Could you check a few things on this model? Use its own coordinates, in mm. A direction names the side the tool comes from. Give positions to 0.01 mm unless a question says otherwise; leave off trailing zeros. Order: outer loops, then holes, each group sorted by start corner. A loop starts at its lowest first (then second) coordinate and runs counter-clockwise, first axis right, second up.
(1) Imagine slicing it at B-B, the plane x = 6. Write out the boundary of the cut face in (y, z).
(2) If I drill on probe 1 along Y at (x, z) = (4.25, 0); probe 2 along Y at (x, z) = (10.3, 0) (3 decimals); probe 3 along X at (y, z) = (0.25, 5), over which ranges is the centre line in solid material (lowest first)?
(3) If we mould it in two halves opening along Z, with no side actions, what happens to faces 4 (the flat face through (10, 2, 2)), 5 (the flat face through (10.8, -5, -5)), 6 (the cylindrical face through (3.94, 1.1, -3.48))? For each: released by +Z, released by -Z, zero draft, split by the parting line, or undercut.
(4) Will these pins go through, and if not, where does the flat tip stop? pin 1 (2 mm diameter, centred on x = 9, y = -6, fed in from -Z); pin 2 (3 mm diameter, centred on x = 1, y = -4.5, fed in from -Z); pin 3 (2 mm diameter, centred on x = 4, y = -3.5, fed in from -Z); pin 4 (3.5 mm diameter, centred on y = 0, z = 0, fed in from +X).
(5) Imagine slicing it at A-A, the plane z = 0. Write out the boundary of the cut face in (x, y) (3 decimals).
(6) On a 3-axis mill with a long thin cutter (end or side, diameter ignored), from which of +Z, -Z, +X, -X, +Y, -Y can I reach the whole of each face in a straight line? I mean faces 1 (the flat face through (8, 0, -4)), 2 (the cylindrical face through (4.93, 0.631, -2.003)), 3 (the cylindrical face through (9.44, 8.38, 3.71)). Say none if no direction works.
from build123d import *

# Parameters (mm, degrees)
SKETCH3_R           = 3.65
SKETCH3_R_2         = 2.1
BOSS_EXTRUDE3_DEPTH = 10
BOSS_EXTRUDE5_START = -2
SKETCH10_R          = 11.275
SKETCH10_R_2        = 3.65
BOSS_EXTRUDE5_DEPTH = 2
SKETCH11_R          = 11.275
SKETCH11_R_2        = 6.775
BOSS_EXTRUDE6_DEPTH = 0.8
SKETCH12_R          = 1
CUT_EXTRUDE2_DEPTH  = 2.75
FILLET3_R           = 1


with BuildPart() as part:
    # Sketch3 → Boss-Extrude3 (new body)
    with BuildSketch(Plane(origin=(0, 0, 0), x_dir=(0, 0, -1), z_dir=(1, 0, 0))):
        Circle(SKETCH3_R)
        Circle(SKETCH3_R_2, mode=Mode.SUBTRACT)
    extrude(amount=BOSS_EXTRUDE3_DEPTH)

    # Sketch10 → Boss-Extrude5 (add)
    with BuildSketch(Plane(origin=(10, 0, 0), x_dir=(0, 0, -1), z_dir=(1, 0, 0)).offset(BOSS_EXTRUDE5_START)):
        Circle(SKETCH10_R)
        Circle(SKETCH10_R_2, mode=Mode.SUBTRACT)
    extrude(amount=BOSS_EXTRUDE5_DEPTH)

    # Sketch11 → Boss-Extrude6 (add)
    with BuildSketch(Plane(origin=(10, 0, 0), x_dir=(0, 0, -1), z_dir=(1, 0, 0))):
        Circle(SKETCH11_R)
        Circle(SKETCH11_R_2, mode=Mode.SUBTRACT)
    extrude(amount=BOSS_EXTRUDE6_DEPTH)

    # Sketch12 → Cut-Extrude2 (cut)
    with BuildSketch(Plane(origin=(10.8, 0, 0), x_dir=(0, 0, -1), z_dir=(1, 0, 0))):
        with BuildLine():
            ThreePointArc((-3.665, -8.080017017), (-3.699074174, -7.821197972), (-3.798974596, -7.580017017))
            Line((-3.798974596, -7.580017017), (-4.665, -8.080017017))
            Line((-4.665, -8.080017017), (-4.665, -7.080017017))
            ThreePointArc((-4.665, -7.080017017), (-5.372106781, -8.787123798), (-3.665, -8.080017017))
        make_face()
        with BuildLine():
            Line((-4.665, -8.080017017), (-3.798974596, -7.580017017))
            ThreePointArc((-3.798974596, -7.580017017), (-4.165, -7.213991614), (-4.665, -7.080017017))
            Line((-4.665, -7.080017017), (-4.665, -8.080017017))
        make_face()
        with BuildLine():
            Line((8.463974596, -0.5), (9.33, 0))
            Line((9.33, 0), (8.463974596, 0.5))
            ThreePointArc((8.463974596, 0.5), (8.33, 0), (8.463974596, -0.5))
        make_face()
        with BuildLine():
            Line((8.463974596, 0.5), (9.33, 0))
            Line((9.33, 0), (8.463974596, -0.5))
            ThreePointArc((8.463974596, -0.5), (9.588819045, -0.965925826), (10.33, 0))
            ThreePointArc((10.33, 0), (9.588819045, 0.965925826), (8.463974596, 0.5))
        make_face()
        with Locations((-4.665, 8.080017017)):
            Circle(SKETCH12_R)
    extrude(amount=-CUT_EXTRUDE2_DEPTH, mode=Mode.SUBTRACT)

    # Fillet3
    fillet3_edges = [part.edges().sort_by_distance(p)[0] for p in [
        (8, 0, 11.275),
    ]]
    fillet(fillet3_edges, radius=FILLET3_R)


solid = part.part
Answer block:
1. outline: circle Ø7.3 at (0, 0); hole circle Ø4.2 at (0, 0)
2. probe 1: y = -3.65 to -2.1, 2.1 to 3.65
2. probe 2: y = -11.275 to -6.775, 6.775 to 11.275
2. probe 3: x = 8 to 10
3. face 4: undercut
3. face 5: zero draft
3. face 6: split by the parting line
4. pin 1: stops at z = -10.11
4. pin 2: stops at z = -2.08
4. pin 3: stops at z = -2.66
4. pin 4: passes through
5. outline: (0, -3.65) - (8, -3.65) - (8, -10.275) arc R1 ccw to (9, -11.275) - (10.8, -11.275) - (10.8, -6.775) - (10, -6.775) - (10, -2.1) - (0, -2.1) - close; (0, 2.1) - (10, 2.1) - (10, 6.775) - (10.8, 6.775) - (10.8, 11.275) - (9, 11.275) arc R1 ccw to (8, 10.275) - (8, 3.65) - (0, 3.65) - close
6. face 1: -X
6. face 2: +X, -X
6. face 3: +X
